Build history of the part. All positions in model axes, mm. Give positions to 0.01 mm unless a question says otherwise; leave off trailing zeros. Order: outer loops, then holes, each group sorted by start corner. A loop starts at its lowest first (then second) coordinate and runs counter-clockwise, first axis right, second up. Notation, with made-up numbers: (68, 53) - (83, 53) arc R37 ccw to (83, 89) - close; hole circle Ø1 at (57, 62). An arc over 180 degrees is marked (long way). Use a Markdown table: item, result. Add a question column.
(1) Slice it at B-B (x = 6). Count the separate pieces of the cut face and the enclosed holes in it, then the cut area to 3 significant figures.
(2) Wall check: line 1 (Y direction, x = 2.75, z = -31); line 2 (Y direction, x = 1, z = -34); line 3 (Z direction, x = 8.5, y = 12). Give the ranges that are in metal, low to high.
(3) Mould opens along Y. For faces 1 (the face through (4.93, 7.46, 23.08)), 2 (the face through (5, -43.694, 0)), 3 (the face through (4.93, -14.9, 87.39)), 4 (the face through (5, -63.694, -61)) say: +Y half, -Y half, draft (parallel to the pull), parting line (faces both ways), or undercut.
(4) Slice it at C-C (z = 71). Write the cut outline in (x, y), then the cut area to 3 significant figures.
(5) Flat gauge pins, fed straight in: pin 1 (3 mm diameter, centred on x = 4, z = 37, fed in from -Y); pin 2 (6 mm diameter, centred on x = 2, z = 59.5, fed in from -Y). Where does each tip first touch, or does it go through?
(6) Slice it at A-A (z = -83). Write the cut outline in (x, y).
from build123d import *

# Parameters (mm, degrees)
SKETCH1_R           = 11.1125
SKETCH1_R_2         = 1.5875
SKETCH1_R_3         = 1.6
BOSS_EXTRUDE1_DEPTH = 10


with BuildPart() as part:
    # Sketch1 → Boss-Extrude1 (new body)
    with BuildSketch(Plane(origin=(0, 0, 0), x_dir=(0, 0, -1), z_dir=(1, 0, 0))):
        with BuildLine():
            Line((-31, -63.693575035), (155, -63.693575035))
            ThreePointArc((155, -63.693575035), (164.363641759, -57.203876021), (161.573840181, -46.158017638))
            Line((161.573840181, -46.158017638), (49.436340181, 51.668057396))
            ThreePointArc((49.436340181, 51.668057396), (46.372800987, 53.496141759), (42.8625, 54.1325))
            Line((42.8625, 54.1325), (-42.8625, 54.1325))
            ThreePointArc((-42.8625, 54.1325), (-47.78371281, 52.83776648), (-51.430593782, 49.288832897))
            Line((-51.430593782, 49.288832897), (-86.068093782, -8.267060862))
            ThreePointArc((-86.068093782, -8.267060862), (-87.375969658, -14.993496721), (-84.046536707, -20.982683219))
            Line((-84.046536707, -20.982683219), (-37.546536707, -61.252864495))
            ThreePointArc((-37.546536707, -61.252864495), (-34.49335837, -63.063550878), (-31, -63.693575035))
        make_face()
        Circle(SKETCH1_R, mode=Mode.SUBTRACT)
        with Locations((-15.4305, 15.4305)):
            Circle(SKETCH1_R_2, mode=Mode.SUBTRACT)
        with Locations((15.4305, 15.4305)):
            Circle(SKETCH1_R_2, mode=Mode.SUBTRACT)
        with Locations((15.4305, -15.4305)):
            Circle(SKETCH1_R_2, mode=Mode.SUBTRACT)
        with Locations((-15.4305, -15.4305)):
            Circle(SKETCH1_R_2, mode=Mode.SUBTRACT)
        with Locations((-77.5, -13.423393759)):
            Circle(SKETCH1_R_3, mode=Mode.SUBTRACT)
        with Locations((-31, -53.693575035)):
            Circle(SKETCH1_R_3, mode=Mode.SUBTRACT)
        with Locations((31, -53.693575035)):
            Circle(SKETCH1_R_3, mode=Mode.SUBTRACT)
        with Locations((93, -53.693575035)):
            Circle(SKETCH1_R_3, mode=Mode.SUBTRACT)
        with Locations((155, -53.693575035)):
            Circle(SKETCH1_R_3, mode=Mode.SUBTRACT)
        with BuildLine():
            Line((33.3375, 47.3075), (42.8625, 47.3075))
            ThreePointArc((42.8625, 47.3075), (46.0375, 44.1325), (42.8625, 40.9575))
            Line((42.8625, 40.9575), (33.3375, 40.9575))
            ThreePointArc((33.3375, 40.9575), (30.1625, 44.1325), (33.3375, 47.3075))
        make_face(mode=Mode.SUBTRACT)
        with BuildLine():
            Line((-33.3375, 47.3075), (-42.8625, 47.3075))
            ThreePointArc((-42.8625, 47.3075), (-46.0375, 44.1325), (-42.8625, 40.9575))
            Line((-42.8625, 40.9575), (-33.3375, 40.9575))
            ThreePointArc((-33.3375, 40.9575), (-30.1625, 44.1325), (-33.3375, 47.3075))
        make_face(mode=Mode.SUBTRACT)
        with BuildLine():
            Line((13.297041151, 34.1325), (-13.297041151, 34.1325))
            ThreePointArc((-13.297041151, 34.1325), (-15.599695746, 32.606040867), (-15.090423831, 29.890725455))
            Line((-15.090423831, 29.890725455), (-1.793382679, 16.1996979))
            ThreePointArc((-1.793382679, 16.1996979), (0, 15.441472444), (1.793382679, 16.1996979))
            Line((1.793382679, 16.1996979), (15.090423831, 29.890725455))
            ThreePointArc((15.090423831, 29.890725455), (15.599695746, 32.606040867), (13.297041151, 34.1325))
        make_face(mode=Mode.SUBTRACT)
        with BuildLine():
            Line((-51.815124471, -22.438391905), (-35.436810722, -36.622427682))
            ThreePointArc((-35.436810722, -36.622427682), (-33.795573215, -37.08283305), (-32.395452573, -36.11056979))
            Line((-32.395452573, -36.11056979), (-21.47657674, -17.198522087))
            ThreePointArc((-21.47657674, -17.198522087), (-21.568587763, -15.053852045), (-23.549955622, -14.22786353))
            Line((-23.549955622, -14.22786353), (-50.847145204, -18.955875456))
            ThreePointArc((-50.847145204, -18.955875456), (-52.43276537, -20.390931102), (-51.815124471, -22.438391905))
        make_face(mode=Mode.SUBTRACT)
        with BuildLine():
            Line((-42.663433079, 25.069654772), (-54.916393111, 4.709349732))
            ThreePointArc((-54.916393111, 4.709349732), (-54.834634818, 2.004177703), (-52.338364397, 0.958580214))
            Line((-52.338364397, 0.958580214), (-25.011725561, 5.798578931))
            ThreePointArc((-25.011725561, 5.798578931), (-23.068694594, 7.492029199), (-23.65434815, 10.002039769))
            Line((-23.65434815, 10.002039769), (-38.728026954, 25.522346093))
            ThreePointArc((-38.728026954, 25.522346093), (-40.807101694, 26.264193912), (-42.663433079, 25.069654772))
        make_face(mode=Mode.SUBTRACT)
        with BuildLine():
            Line((-11.514428415, -39.943575035), (-2.165063509, -23.75))
            ThreePointArc((-2.165063509, -23.75), (0, -22.5), (2.165063509, -23.75))
            Line((2.165063509, -23.75), (11.514428415, -39.943575035))
            ThreePointArc((11.514428415, -39.943575035), (11.514428415, -42.443575035), (9.349364905, -43.693575035))
            Line((9.349364905, -43.693575035), (-9.349364905, -43.693575035))
            ThreePointArc((-9.349364905, -43.693575035), (-11.514428415, -42.443575035), (-11.514428415, -39.943575035))
        make_face(mode=Mode.SUBTRACT)
        with BuildLine():
            Line((38.216878365, -43.693575035), (46.349364905, -43.693575035))
            ThreePointArc((46.349364905, -43.693575035), (48.764179471, -41.840622647), (47.599364905, -39.028511525))
            Line((47.599364905, -39.028511525), (35.400635095, -31.985571585))
            ThreePointArc((35.400635095, -31.985571585), (32.382868142, -32.382868142), (31.985571585, -35.400635095))
            Line((31.985571585, -35.400635095), (36.051814855, -42.443575035))
            ThreePointArc((36.051814855, -42.443575035), (36.966878365, -43.358638544), (38.216878365, -43.693575035))
        make_face(mode=Mode.SUBTRACT)
        with BuildLine():
            Line((47.00332879, 27.249721463), (90.259443654, -10.48587937))
            ThreePointArc((90.259443654, -10.48587937), (91.29812152, -16.761486275), (85.335889386, -18.978213981))
            Line((85.335889386, -18.978213981), (25.545919003, 1.733639317))
            ThreePointArc((25.545919003, 1.733639317), (22.317964542, 5.302436868), (23.59578782, 9.941744319))
            Line((23.59578782, 9.941744319), (40.12964334, 26.965491854))
            ThreePointArc((40.12964334, 26.965491854), (43.509833256, 28.4776736), (47.00332879, 27.249721463))
        make_face(mode=Mode.SUBTRACT)
    extrude(amount=BOSS_EXTRUDE1_DEPTH)


solid = part.part
Solution:
| question | item | result |
|---|---|---|
| 1 | separate pieces | 1 |
| 1 | enclosed holes | 18 |
| 1 | area | 17,400 mm2 |
| 2 | line 1 | -63.69 to -55.29, -52.09 to -0.16, 17.57 to 41.98, 46.28 to 54.13 |
| 2 | line 2 | -63.69 to -38.89, -31.66 to -1.19, 20.65 to 40.96, 47.31 to 54.13 |
| 2 | line 3 | -94.91 to -64.48, -25.59 to 25.59, 50.53 to 73.87 |
| 3 | face 1 | undercut |
| 3 | face 2 | undercut |
| 3 | face 3 | parting line |
| 3 | face 4 | -Y half |
| 4 | outline | (0, -32.28) - (10, -32.28) - (10, 16.77) - (0, 16.77) - close |
| 4 | area | 491 mm2 |
| 5 | pin 1 | y = -62.62 |
| 5 | pin 2 | y = -44.84 |
| 6 | outline | (0, -63.69) - (10, -63.69) - (10, -18.17) - (0, -18.17) - close; (0, -4.15) - (10, -4.15) - (10, 22.39) - (0, 22.39) - close |
